```python
from build123d import *

# Parameters (mm, degrees)
BOSS_EXTRUDE1_DEPTH     = 20
SHELL1_T                = 3
CUT_EXTRUDE1_REACH      = 175.853
SKETCH4_W               = 15
SKETCH4_H               = 25
CUT_EXTRUDE2_DEPTH      = 178.270979012
CUT_EXTRUDE3_REACH      = 175.853
SKETCH5_W               = 12
SKETCH5_H               = 25
SKETCH6_R               = 6
CUT_EXTRUDE4_DEPTH      = 166.435788148
CUT_EXTRUDE5_REACH      = 175.853
CUT_EXTRUDE5_END_RADIUS = 149.692307692
SKETCH7_W               = 15
SKETCH7_H               = 33
FILLET1_R               = 2
FILLET2_R               = 1


with BuildPart() as part:
    # Sketch2 → Boss-Extrude1 (new, symmetric)
    with BuildSketch(Plane(origin=(0, 0, 0), x_dir=(1, 0, 0), z_dir=(0, 1, 0))):
        with BuildLine():
            Line((65, 0), (65, 75))
            ThreePointArc((65, 75), (38.25588773, 93.89935692), (28, 125))
            Line((28, 125), (28, 160))
            Line((28, 160), (0, 160))
            Line((0, 160), (0, 125))
            ThreePointArc((0, 125), (17.221126888, 54.554985982), (65, 0))
        make_face()
    extrude(amount=BOSS_EXTRUDE1_DEPTH, both=True)

    # Shell1 (no face opened: a closed hollow body)
    add(offset(amount=-SHELL1_T, mode=Mode.PRIVATE), mode=Mode.SUBTRACT)

    # Sketch3 → Cut-Extrude1 (cut, up to next)
    with BuildSketch(Plane(origin=(65, 0, 0), x_dir=(0, 0, -1), z_dir=(1, 0, 0)), mode=Mode.PRIVATE) as cut_extrude1_sk1:
        with BuildLine():
            Line((12.5, 4), (62.5, 4))
            ThreePointArc((62.5, 4), (66.5, 0), (62.5, -4))
            Line((62.5, -4), (12.5, -4))
            ThreePointArc((12.5, -4), (8.5, 0), (12.5, 4))
        make_face()
    cut_extrude1_tool1 = extrude(cut_extrude1_sk1.sketch, amount=-CUT_EXTRUDE1_REACH, mode=Mode.PRIVATE) & part.part
    add(cut_extrude1_tool1.solids().sort_by_distance((65, 0, -37.5))[0], mode=Mode.SUBTRACT)

    # Sketch4 → Cut-Extrude2 (cut, through all)
    with BuildSketch(Plane(origin=(0, 20, 0), x_dir=(1, 0, 0), z_dir=(0, 1, 0))):
        with Locations((14, 140.5)):
            Rectangle(SKETCH4_W, SKETCH4_H)
    extrude(amount=-CUT_EXTRUDE2_DEPTH, mode=Mode.SUBTRACT)

    # Sketch5 → Cut-Extrude3 (cut, up to next)
    with BuildSketch(Plane(origin=(0, 0, -160), x_dir=(-1, 0, 0), z_dir=(0, 0, -1)), mode=Mode.PRIVATE) as cut_extrude3_sk1:
        with Locations((-14, 0)):
            Rectangle(SKETCH5_W, SKETCH5_H)
    cut_extrude3_tool1 = extrude(cut_extrude3_sk1.sketch, amount=-CUT_EXTRUDE3_REACH, mode=Mode.PRIVATE) & part.part
    add(cut_extrude3_tool1.solids().sort_by_distance((14, 0, -160))[0], mode=Mode.SUBTRACT)

    # Sketch6 → Cut-Extrude4 (cut, through all)
    with BuildSketch(Plane(origin=(28, 0, 0), x_dir=(0, 0, -1), z_dir=(1, 0, 0))):
        with Locations((142.5, 0)):
            Circle(SKETCH6_R)
    extrude(amount=-CUT_EXTRUDE4_DEPTH, mode=Mode.SUBTRACT)

    # Cut-Extrude5: up to this cylinder (the profile starts outside it)
    cut_extrude5_end = Plane(origin=(152.692307692, 0, -125), z_dir=(0, -1, 0)) * Cylinder(CUT_EXTRUDE5_END_RADIUS, 652.090615385, mode=Mode.PRIVATE)
    # Sketch7 → Cut-Extrude5 (cut, up to the surface)
    with BuildSketch(Plane.XY, mode=Mode.PRIVATE) as cut_extrude5_sk1:
        with Locations((54.5, 0)):
            Rectangle(SKETCH7_W, SKETCH7_H)
    cut_extrude5_tool1 = extrude(cut_extrude5_sk1.sketch, amount=-CUT_EXTRUDE5_REACH, mode=Mode.PRIVATE) - cut_extrude5_end
    add(cut_extrude5_tool1.solids().sort_by_distance((54.5, 0, 0))[0], mode=Mode.SUBTRACT)

    # Fillet1
    # the kernel refuses this fillet: 2 mm, written as the material it takes off along each edge
    with BuildSketch(Plane(origin=(65, -29.832655727, 0), x_dir=(-0.8111753720748651, 0, -0.584802971725695), z_dir=(0, 1, 0))) as fillet1_piece_1:
        with BuildLine():
            CenterArc((3.9073042, -1.999834123), FILLET1_R, 89.26206466, 126.527007428)
            Line((2.284953456, -3.169440067), (0, 0))
            ThreePointArc((0, 0), (1.966531145, 0.012664047), (3.933062291, 0))
        make_face()
    extrude(amount=59.665311453, mode=Mode.SUBTRACT)

    # Fillet2
    fillet2_edges = [part.edges().sort_by_distance(p)[0] for p in [
        (38.25588773, 20, -93.89935692),
        (0, 0, -160),
        (28, 0, -160),
        (65, 0, -75),
        (65, -20, -39.453609648),
        (65, 20, -39.453609648),
        (63.899775935, -20, -2.121049297),
        (63.899775935, 20, -2.121049297),
        (28, 20, -142.5),
        (14, 20, -160),
        (0, 20, -142.5),
        (16.325098118, 20, -56.305568047),
        (21.5, -20, -140.5),
        (14, -20, -128),
        (6.5, -20, -140.5),
        (14, -20, -153),
        (21.5, 20, -140.5),
        (14, 20, -153),
        (6.5, 20, -140.5),
        (14, 20, -128),
        (0, -20, -142.5),
        (14, -20, -160),
        (28, -20, -142.5),
        (38.25588773, -20, -93.89935692),
        (16.325098118, -20, -56.305568047),
    ]]
    fillet(fillet2_edges, radius=FILLET2_R)


solid = part.part
```
The model under review builds one solid part; all positions refer to its coordinate system, in mm. A direction names the side the tool comes from. Coordinates: 2 decimals unless noted, no trailing zeros. Write each loop counter-clockwise with the first axis right and the second up, starting at its lowest first coordinate (ties: lowest second). Pieces come first, ordered by that corner, then holes.
1) The part is to be moulded in two halves that separate along X. For faces 5 (the face through (38.314, 0.266, -93.821)), 6 (the face through (63.872, -0.266, -2.107)), 7 (the face through (20, 0, -159)), 8 (the face through (63.5, -0.1, -8.5)), say which applies: pulls with the +X half, pulls with the -X half, needs draft (parallel to the pull), parting line crosses it, or undercut.
2) Clearance check with flat-ended pins moving along their axes: pin 1 Ø10 at (y, z) = (13, -83.5) entering from -X; pin 2 Ø6.5 at (x, y) = (12.5, 4) entering from +Z; pin 3 Ø10 at (x, y) = (39.5, 13.5) entering from +Z. State where each tip first meets the part, or that it passes through.
3) We need section B-B on y = -14.5. State the section outline as (x, z) points.
4) To check wall thickness, follow probe 1 along Y at (x, z) = (41, -26); probe 2 along Y at (x, z) = (26, -142); probe 3 along X at (y, z) = (-13, -67.5). State the ranges of each line that lie inside material, in increasing order.
5) We need section A-A on z = -145. Count the separate pieces of the cut face and the enclosed holes in it, then the cut area to 3 significant figures.
6) Machinability: for faces 1 (the face through (28, 4.5, -138)), 2 (the face through (8, 0, -159)), 3 (the face through (54, -16.5, -11)), 4 (the face through (7, 0, -157)), which of the approach directions +Z, -Z, +X, -X, +Y, -Y give a long, thin tool a straight path to every point of the face, cutting with its end or side? Answer none if there is none.
Answer list:
1. face 5: pulls with the +X half
1. face 6: parting line crosses it
1. face 7: undercut
1. face 8: needs draft
2. pin 1: stops at x = 4.43
2. pin 2: stops at z = -57.46
2. pin 3: stops at z = -17.25
3. outline: (0, -159) arc R1 ccw to (1, -160) - (27, -160) arc R1 ccw to (28, -159) - (28, -125) arc R52.28 cw to (64.31, -75.22) arc R1 ccw to (65, -74.27) - (65, -3.91) arc R2 ccw to (62, -2.18) - (62, -72.83) arc R55.28 ccw to (25, -125) - (25, -157) - (3, -157) - (3, -125) arc R149.69 cw to (47, -19) - (47, -14.8) arc R152.69 ccw to (0, -125) - close
4. probe 1: y = -20 to -17, 17 to 20
4. probe 2: y = -20 to -5.98, 5.98 to 20
4. probe 3: x = 11.24 to 14.48, 62 to 65
5. separate pieces: 4
5. enclosed holes: 0
5. area: 215 mm2
6. face 1: -Z, +X, +Y, -Y
6. face 2: -Z
6. face 3: +Z
6. face 4: none
